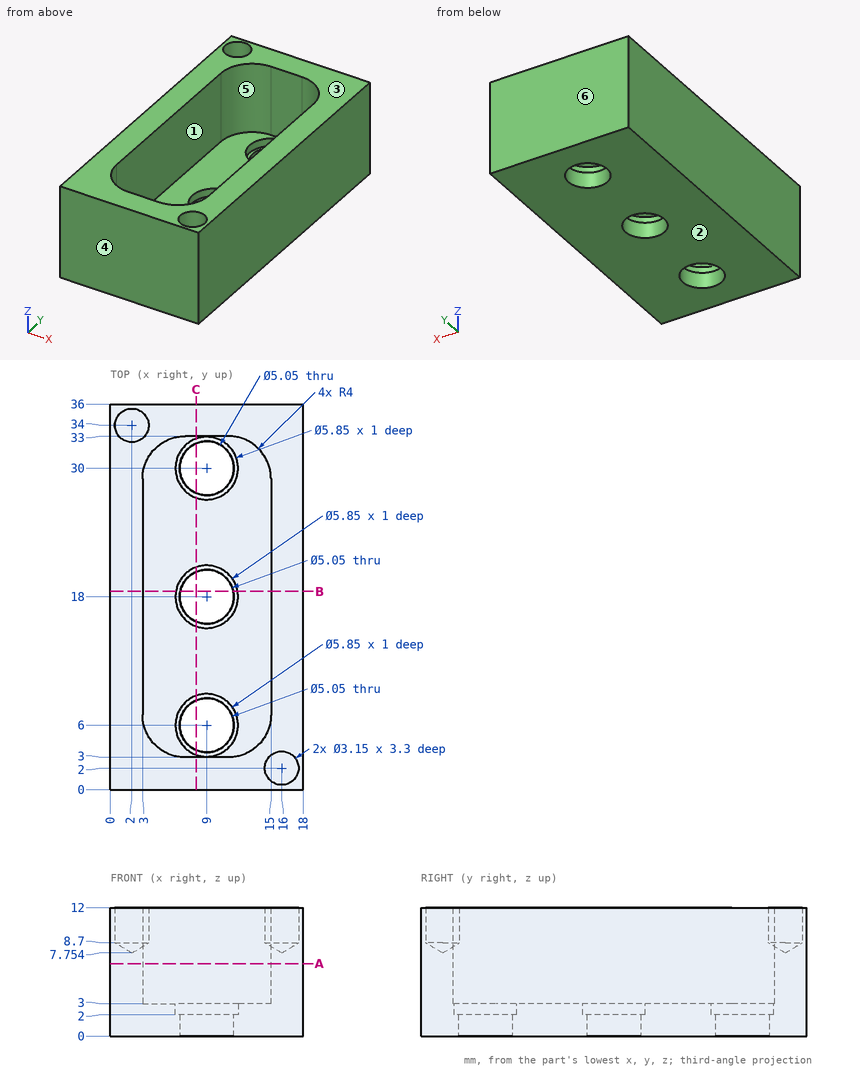
Could you check a few things on this drawing? It's one solid part, dimensions in mm from its lowest x, y, z. A direction names the side the tool comes from. Coordinates: 2 decimals unless noted, no trailing zeros. Write each loop counter-clockwise with the first axis right and the second up, starting at its lowest first coordinate (ties: lowest second). Pieces come first, ordered by that corner, then holes.
Q1. Please list where these lines run through material, in increasing order: L1, parallel to Y at x = 9, z = 2.7 (1 decimal); L2, parallel to X at y = 6, z = 1 (1 decimal); L3, parallel to X at y = 14.5, z = 8.75.
Results found:
L1: y = 0 to 3.1, 8.9 to 15.1, 20.9 to 27.1, 32.9 to 36
L2: x = 0 to 6.5, 11.5 to 18
L3: x = 0 to 3, 15 to 18
Q2. Imagine slicing it at A-A, the plane z = 6.75. List the corners of the cut face in (x, y) for me.
Results found:
outline: (0, 0) - (18, 0) - (18, 36) - (0, 36) - close; hole (3, 7) arc R4 ccw to (7, 3) - (11, 3) arc R4 ccw to (15, 7) - (15, 29) arc R4 ccw to (11, 33) - (7, 33) arc R4 ccw to (3, 29) - close
Q3. Which directions (+Z, -Z, +X, -X, +Y, -Y) give clear straight access to the entire face, cutting with the end or side of a thin tool? Please do the marked faces 1 and 2.
Results found:
face 1: +Z
face 2: -Z, +X, -X, +Y, -Y
Q4. Imagine slicing it at C-C, the plane x = 8. Count the separate pieces of the cut face and the enclosed holes in it, plus the area to 3 significant figures.
Results found:
separate pieces: 4
enclosed holes: 0
area: 118 mm2
Q5. If we mould it in two halves opening along Y, with no side actions, what happens to the marked faces 3, 4, 5 and 6? For each: +Y half, -Y half, draft (parallel to the pull), parting line (faces both ways), or undercut.
Results found:
face 3: draft
face 4: -Y half
face 5: undercut
face 6: +Y half
Q6. Imagine slicing it at B-B, the plane y = 18.5. List the corners of the cut face in (x, z) for me (1 decimal).
Results found:
outline: (0, 0) - (6.5, 0) - (6.5, 2) - (6.1, 2) - (6.1, 3) - (3, 3) - (3, 12) - (0, 12) - close; (11.5, 0) - (18, 0) - (18, 12) - (15, 12) - (15, 3) - (11.9, 3) - (11.9, 2) - (11.5, 2) - close
Q7. For P1, Ø1.9, axis at x = 2, y = 34, coming from the +Z side (1 decimal); P2, Ø6, axis at x = 9.5, y = 17.5, coming from the +Z side, each with a flat end and sliding along its axis, tell me the tip position at first contact or that it passes through.
Results found:
P1: stops at z = 8.3
P2: stops at z = 3
